from build123d import *

# Parameters (mm, degrees)
AUFSATZ_LINEAR_START             = -2.5
AUFSATZ_LINEAR_AUSTRAGEN1_DEPTH  = 6
VERRUNDUNG1_R                    = 1
F_2_5_2_5_DURCHMESSER_BOHRUNG1_D = 2.5


with BuildPart() as part:
    # Skizze1 → Aufsatz-Linear austragen1 (new body)
    with BuildSketch(Plane.XY.offset(AUFSATZ_LINEAR_START)):
        with BuildLine():
            Line((225, 17), (409.023823037, 17))
            ThreePointArc((409.023823037, 17), (413.907829989, 21.680453509), (419.801960973, 25))
            Line((419.801960973, 25), (10.198039027, 25))
            ThreePointArc((10.198039027, 25), (16.092170011, 21.680453509), (20.976176963, 17))
            Line((20.976176963, 17), (225, 17))
        make_face()
    extrude(amount=-AUFSATZ_LINEAR_AUSTRAGEN1_DEPTH)

    # Verrundung1
    verrundung1_edges = [part.edges().sort_by_distance(p)[0] for p in [
        (409.023823037, 17, -5.5),
        (20.976176963, 17, -5.5),
        (10.198039027, 25, -5.5),
        (419.801960973, 25, -5.5),
    ]]
    fillet(verrundung1_edges, radius=VERRUNDUNG1_R)

    # Ø2.5 (2.5) Durchmesser Bohrung1 (through all)
    with Locations(Plane.XY.offset(-2.5)):
        with Locations((400, 21), (330, 21), (260, 21), (190, 21), (120, 21), (50, 21)):
            Hole(F_2_5_2_5_DURCHMESSER_BOHRUNG1_D / 2)


solid = part.part
Source: CAD feature listing. Evaluate the final solid. Frame: model axes, mm. Give positions to 0.01 mm unless a question says otherwise; leave off trailing zeros. Write each loop counter-clockwise with the first axis right and the second up, starting at its lowest first coordinate (ties: lowest second). Pieces come first, ordered by that corner, then holes. Notation, with made-up numbers: M 88,41.25 L 93,41.25 A18 ccw 93,67.25 Z; hole C 22.25,33 d9. An arc over 180 degrees is marked long. Return JSON: item names as keys, results as strings. Group by question number.
1) Cut plane A-A, the plane z = -5.6. Output: boundary loops of the cut face in (x, y).
2) Pin query (flat end, axial travel): P1, Ø1.5, axis at y = 19, z = -5.5, coming from the +X side; P2, Ø1.5, axis at x = 190, y = 21, coming from the -Z side; P3, Ø2, axis at y = 20.5, z = -5.5, coming from the +X side. Return the tip coordinate at first contact, or that it passes through.
3) Material intervals for line 1 along Y through (x, z) = (330, -5.95); line 2 along X through (y, z) = (23.25, -4.35); line 3 along X through (y, z) = (18.25, -3.3), sorted ascending. Write a range as [from, to].
4) Cut plane B-B, the plane y = 21. Output: boundary loops of the cut face in (x, z), plus the area to 3 significant figures.
Recorded:
{
 "1": {"outline": "M 13.91,23.14 A27 cw 20.68,17.36 A1 ccw 21.45,17 L 408.55,17 A1 ccw 409.32,17.36 A27 cw 416.09,23.14 A1 ccw 415.58,25 L 14.42,25 A1 ccw Z; hole C 50,21 d2.5; hole C 120,21 d2.5; hole C 190,21 d2.5; hole C 260,21 d2.5; hole C 330,21 d2.5; hole C 400,21 d2.5"},
 "2": {"P1": "stops at x = 411.59", "P2": "passes through", "P3": "stops at x = 413.67"},
 "3": {"line 1": "y = [17, 19.75], [22.25, 25]", "line 2": "x = [13.76, 416.24]", "line 3": "x = [19.9, 410.1]"},
 "4": {"outline": "M 16.97,-8.5 L 48.75,-8.5 L 48.75,-2.5 L 16.97,-2.5 Z; M 51.25,-8.5 L 118.75,-8.5 L 118.75,-2.5 L 51.25,-2.5 Z; M 121.25,-8.5 L 188.75,-8.5 L 188.75,-2.5 L 121.25,-2.5 Z; M 191.25,-8.5 L 258.75,-8.5 L 258.75,-2.5 L 191.25,-2.5 Z; M 261.25,-8.5 L 328.75,-8.5 L 328.75,-2.5 L 261.25,-2.5 Z; M 331.25,-8.5 L 398.75,-8.5 L 398.75,-2.5 L 331.25,-2.5 Z; M 401.25,-8.5 L 413.03,-8.5 L 413.03,-2.5 L 401.25,-2.5 Z", "area": "2,290 mm²"}
}
